Verification items for this drawing (mm, ordinates from the low corner). A direction names the side the tool comes from. Coordinates: 2 decimals unless noted, no trailing zeros. Write each loop counter-clockwise with the first axis right and the second up, starting at its lowest first coordinate (ties: lowest second). Pieces come first, ordered by that corner, then holes. Notation, with made-up numbers: (13.5, 4.25) -> (48.5, 4.25) arc R27 ccw to (48.5, 41.25) -> close; hole circle Ø7 at (30, -12). An arc over 180 degrees is marked (long way). One line per question, with ' | ' between items.
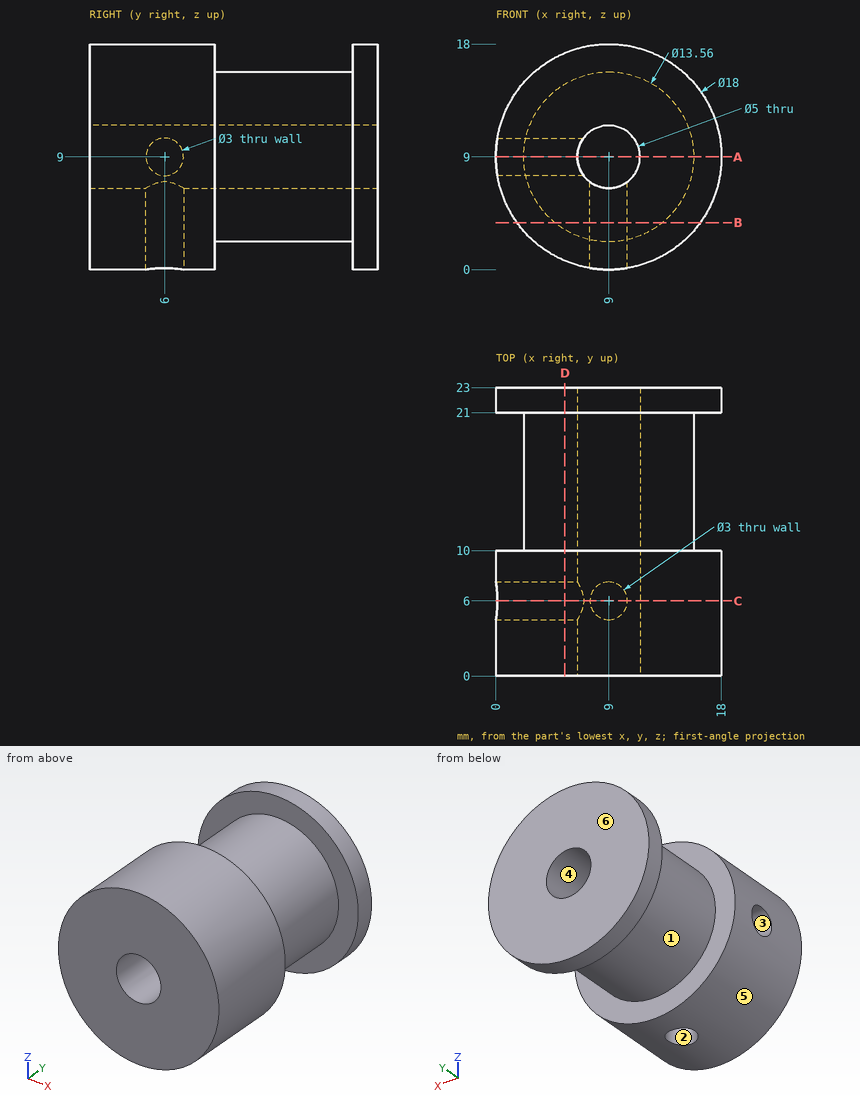
(1) Cross-section at A-A (z = 9). Record the cut outline in (x, y), plus the area to 3 significant figures.
Answers below:
outline: (0, 0) -> (6.5, 0) -> (6.5, 4.5) -> (0, 4.5) -> close; (0, 7.5) -> (6.5, 7.5) -> (6.5, 23) -> (0, 23) -> (0, 21) -> (2.22, 21) -> (2.22, 10) -> (0, 10) -> close; (11.5, 0) -> (18, 0) -> (18, 10) -> (15.78, 10) -> (15.78, 21) -> (18, 21) -> (18, 23) -> (11.5, 23) -> close | area: 231 mm²
(2) Material ranges on line 1 (Y direction, x = 1, z = 9); line 2 (Y direction, x = 5, z = 9); line 3 (X direction, y = 8.25, z = 9), recorded low to high.
Answers below:
line 1: y = 0 to 4.5, 7.5 to 10, 21 to 23 | line 2: y = 0 to 4.5, 7.5 to 23 | line 3: x = 0 to 6.5, 11.5 to 18
(3) Tool access check on the marked faces 1, 2 and 3. Record the directions out of +Z, -Z, +X, -X, +Y, -Y that give a thin tool (end or side, any length) a straight path to the whole face; none if there is none.
Answers below:
face 1: none | face 2: -Z | face 3: -X
(4) Cross-section at C-C (y = 6). Record the cut outline in (x, z), plus the area to 3 significant figures.
Answers below:
outline: (0.13, 7.5) arc R9 ccw to (7.5, 0.13) -> (7.5, 7) arc R2.5 cw to (7, 7.5) -> close; (0.13, 10.5) -> (7, 10.5) arc R2.5 cw (long way) to (10.5, 7) -> (10.5, 0.13) arc R9 ccw (long way) to start | area: 195 mm²
(5) Depth check by flat-ended pin: P1, Ø4, axis at x = 14.5, y = 19.5, coming from the +Z side; P2, Ø1, axis at x = 5.5, y = 9.5, coming from the +Z side; P3, Ø1, axis at y = 6.5, z = 16, coming from the -X side. Enter the tip coordinate at first touch or a pass-through.
Answers below:
P1: stops at z = 16.97 | P2: stops at z = 17.49 | P3: stops at x = 2.78
(6) Draft check along Z on the marked faces 4, 5 and 6. Enter one of: pulls with the +Z half, pulls with the -Z half, needs draft (parallel to the pull), parting line crosses it, or undercut.
Answers below:
face 4: undercut | face 5: parting line crosses it | face 6: needs draft
(7) Cross-section at D-D (x = 5.5). Record the cut outline in (y, z).
Answers below:
outline: (0, 0.71) -> (10, 0.71) -> (10, 3.19) -> (21, 3.19) -> (21, 0.71) -> (23, 0.71) -> (23, 17.29) -> (21, 17.29) -> (21, 14.81) -> (10, 14.81) -> (10, 17.29) -> (0, 17.29) -> close; hole circle Ø3 at (6, 9)
(8) Cross-section at B-B (z = 3.75). Record the cut outline in (x, y), plus the area to 3 significant figures.
Answers below:
outline: (1.69, 0) -> (16.31, 0) -> (16.31, 10) -> (13.29, 10) -> (13.29, 21) -> (16.31, 21) -> (16.31, 23) -> (1.69, 23) -> (1.69, 21) -> (4.71, 21) -> (4.71, 10) -> (1.69, 10) -> close; hole circle Ø3 at (9, 6) | area: 263 mm²
